```python
from build123d import *

# Parameters (mm, degrees)
CUT_EXTRUDE_1_DEPTH = 20


with BuildPart() as part:
    # 草图1 → 旋转2 (revolve)
    with BuildSketch(Plane.XY):
        Polygon((-10.868417819, 98.635802469), (-13.209567901, 98.635802469), (-28.575, 15.835802469), (-28.575, 12.835802469), (-43.313271605, 12.835802469), (-43.313271605, 0.635802469), (-36.5, -3.297841726), (-36.5, -7.430553336), (-43.313271605, -11.364197531), (-43.313271605, -17.164197531), (-30, -17.164197531), (-30, -67.164197531), (-20.5, -67.164197531), (-16, -31.164197531), (0, -31.164197531), (0, 25.628046603), (-9.486874299, 31.105296033), (-9.486874299, 45.695475602), (-10.727694805, 46.411863655), (-10.727694805, 88.230958782), (-10.5, 96.54970542), (-10.5, 97.997684089), align=None)
    revolve(axis=Axis((0, 104.892592593, 0), (0, -1, 0)))

    # 草图3 → 切除-拉伸1 (cut)
    with BuildSketch(Plane.XY.offset(50)):
        with BuildLine():
            Line((-9, 12.835802469), (-9, 0.635802469))
            ThreePointArc((-9, 0.635802469), (0, -9.022430093), (9, 0.635802469))
            Line((9, 0.635802469), (9, 12.835802469))
            Line((9, 12.835802469), (-9, 12.835802469))
        make_face()
    cut_extrude_1 = extrude(amount=-CUT_EXTRUDE_1_DEPTH, mode=Mode.SUBTRACT)

    # 镜向1: 切除-拉伸1 across plane
    add(cut_extrude_1.mirror(Plane.XY), mode=Mode.SUBTRACT)


solid = part.part
```
Build history of the part. All positions in model axes, mm. A direction names the side the tool comes from. Coordinates: 2 decimals unless noted, no trailing zeros. Order: outer loops, then holes, each group sorted by start corner. A loop starts at its lowest first (then second) coordinate and runs counter-clockwise, first axis right, second up. Notation, with made-up numbers: M 88,-32 L 99,-32 A25 cw 99,0 Z; hole C 12,65 d2. An arc over 180 degrees is marked long. One line per question, with ' | ' between items. Start each with the question number.
1. Wall check: line 1 along X through (y, z) = (97, 0); line 2 along Y through (x, z) = (-10, -39); line 3 along X through (y, z) = (74, -8). Give the ranges that are in metal, low to high. Write a range as [from, to].
2. Flat gauge pins, fed straight in: P1, Ø11.5, axis at x = 0, z = 0, coming from the -Y side; P2, Ø10, axis at y = 5.5, z = 35, coming from the -X side; P3, Ø13.5, axis at y = 7.5, z = -39, coming from the +X side. Where does each tip first touch, or does it go through?
3. Mould opens along Z. For faces 1 (the face through (-36.493, -5.393, 0.731)), 2 (the face through (2.33, 67.61, 10.47)), 3 (the face through (-1, 12.836, -29)) say: +Z half, -Z half, draft (parallel to the pull), parting line (faces both ways), or undercut.
4. Cut at B-B (y = -13.5). Write the cut outline in (x, z).
5. Cut at C-C (y = 38.5). Write the cut outline in (x, z).
6. Tool access for faces 4 (the face through (28.547, 14.315, -1.256)), 5 (the face through (-9, 7, -36)), 6 (the face through (36.493, -5.393, -0.731)), 7 (the face through (-9, -17.164, -29)), 8 (the face through (-37, -3, 1)): list every direction of +Z, -Z, +X, -X, +Y, -Y with a clear straight run to the whole face (end or side of a thin tool).
7. Cut at A-A (y = -46.5). Write the cut outline in (x, z), plus the area to 3 significant figures.
The answers:
1) line 1: x = [-13.51, -10.5], [10.5, 13.51] | line 2: y = [-17.16, -9.6], [-1.13, 12.84] | line 3: x = [-15.88, -7.15], [7.15, 15.88]
2) P1: stops at y = -31.16 | P2: stops at x = -31.24 | P3: stops at x = 28.91
3) face 1: parting line | face 2: undercut | face 3: draft
4) outline: C 0,0 d86.63
5) outline: C 0,0 d48.74; hole C 0,0 d18.97
6) face 4: +Y | face 5: -Z, +Y | face 6: +X | face 7: -Y | face 8: -X
7) outline: C 0,0 d60; hole C 0,0 d35.83 | area: 1,820 mm2
